Verification items for the finished model (mm, model axes). Coordinates: 2 decimals unless noted, no trailing zeros. Order: outer loops, then holes, each group sorted by start corner. A loop starts at its lowest first (then second) coordinate and runs counter-clockwise, first axis right, second up. Notation, with made-up numbers: (34.25, 63.25) - (68.25, 63.25) arc R31 ccw to (68.25, 100.25) - close; hole circle Ø3 at (71, 84). An arc over 180 degrees is marked (long way). Answer as CSV lines item,"result". Start each with the question number.
1. Material ranges on L1, parallel to Y at x = 0, z = 153.95; L2, parallel to Y at x = 10.5, z = 153.15; L3, parallel to X at y = 37, z = 152.7, recorded low to high. Write a range as [from, to].
2. Section check C-C (x = 7). Record the cut outline in (y, z), and give its area (3 significant figures).
3. Section check B-B (y = -9.5). Record the cut outline in (x, z).
4. Go/stop test with a flat-tipped pin: pin 1 (5 mm diameter, centred on x = 0, y = -41.63, fed in from -Z). Record where the tip stops, or that it passes through.
5. Section check D-D (z = 154.45). Count the separate pieces of the cut face and the enclosed holes in it, and give its area (3 significant figures).
6. Section check A-A (x = -37.5). Record the cut outline in (y, z).
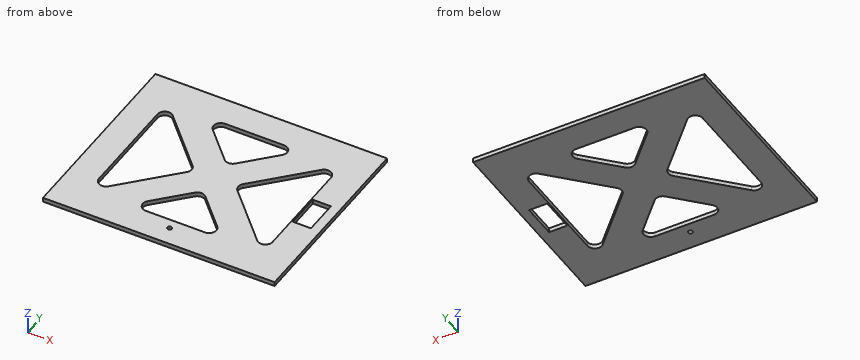
from build123d import *

# Parameters (mm, degrees)
SKETCH1_W           = 160
SKETCH1_H           = 135
BOSS_EXTRUDE1_DEPTH = 3
CUT_EXTRUDE1_DEPTH  = 20
SKETCH3_W           = 10
SKETCH3_H           = 20.2
CUT_EXTRUDE2_DEPTH  = 10
SKETCH5_W           = 10
SKETCH5_H           = 3
BOSS_EXTRUDE2_DEPTH = 30
SKETCH6_W           = 10
SKETCH6_H           = 20.15
CUT_EXTRUDE3_DEPTH  = 30
SKETCH7_W           = 10
SKETCH7_H           = 3
BOSS_EXTRUDE3_DEPTH = 30
SKETCH8_W           = 11.5
SKETCH8_H           = 21.5
CUT_EXTRUDE4_DEPTH  = 10
SKETCH9_W           = 11.5
SKETCH9_H           = 3
BOSS_EXTRUDE5_DEPTH = 30
SKETCH10_W          = 11
SKETCH10_H          = 21
CUT_EXTRUDE5_DEPTH  = 30
SKETCH11_W          = 3
SKETCH11_H          = 21
CUT_EXTRUDE6_DEPTH  = 1.5
SKETCH12_W          = 12.5
SKETCH12_H          = 3
CUT_EXTRUDE7_DEPTH  = 3


with BuildPart() as part:
    # Sketch1 → Boss-Extrude1 (new body)
    with BuildSketch(Plane.XY.offset(152)):
        with Locations((0, 12.91714511)):
            Rectangle(SKETCH1_W, SKETCH1_H)
        with BuildLine():
            Line((-60, -22.204596664), (-60, 48.038886885))
            ThreePointArc((-60, 48.038886885), (-56.872665603, 52.674954566), (-51.402750584, 51.511608676))
            Line((-51.402750584, 51.511608676), (-17.49683417, 16.389866902))
            ThreePointArc((-17.49683417, 16.389866902), (-16.094083586, 12.91714511), (-17.49683417, 9.444423319))
            Line((-17.49683417, 9.444423319), (-51.402750584, -25.677318456))
            ThreePointArc((-51.402750584, -25.677318456), (-56.872665603, -26.840664345), (-60, -22.204596664))
        make_face(mode=Mode.SUBTRACT)
        with BuildLine():
            Line((20.424315219, 60.41714511), (-20.424315219, 60.41714511))
            ThreePointArc((-20.424315219, 60.41714511), (-25.026684661, 57.371165459), (-24.021564635, 51.944423319))
            Line((-24.021564635, 51.944423319), (-3.597249416, 30.787716735))
            ThreePointArc((-3.597249416, 30.787716735), (0, 29.260438526), (3.597249416, 30.787716735))
            Line((3.597249416, 30.787716735), (24.021564635, 51.944423319))
            ThreePointArc((24.021564635, 51.944423319), (25.026684661, 57.371165459), (20.424315219, 60.41714511))
        make_face(mode=Mode.SUBTRACT)
        with BuildLine():
            Line((51.402750584, 51.511608676), (17.49683417, 16.389866902))
            ThreePointArc((17.49683417, 16.389866902), (16.094083586, 12.91714511), (17.49683417, 9.444423319))
            Line((17.49683417, 9.444423319), (51.402750584, -25.677318456))
            ThreePointArc((51.402750584, -25.677318456), (56.872665603, -26.840664345), (60, -22.204596664))
            Line((60, -22.204596664), (60, 48.038886885))
            ThreePointArc((60, 48.038886885), (56.872665603, 52.674954566), (51.402750584, 51.511608676))
        make_face(mode=Mode.SUBTRACT)
        with BuildLine():
            Line((-24.021564635, -26.110133098), (-3.597249416, -4.953426514))
            ThreePointArc((-3.597249416, -4.953426514), (0, -3.426148305), (3.597249416, -4.953426514))
            Line((3.597249416, -4.953426514), (24.021564635, -26.110133098))
            ThreePointArc((24.021564635, -26.110133098), (25.026684661, -31.536875238), (20.424315219, -34.58285489))
            Line((20.424315219, -34.58285489), (-20.424315219, -34.58285489))
            ThreePointArc((-20.424315219, -34.58285489), (-25.026684661, -31.536875238), (-24.021564635, -26.110133098))
        make_face(mode=Mode.SUBTRACT)
    extrude(amount=BOSS_EXTRUDE1_DEPTH)

    # Sketch2 → Cut-Extrude1 (cut)
    with BuildSketch(Plane.XY.offset(155)):
        with BuildLine():
            ThreePointArc((1.5, -41.631936217), (0, -40.131936217), (-1.5, -41.631936217))
            Line((-1.5, -41.631936217), (1.5, -41.631936217))
        make_face()
        with BuildLine():
            Line((1.5, -41.631936217), (-1.5, -41.631936217))
            ThreePointArc((-1.5, -41.631936217), (0, -43.131936217), (1.5, -41.631936217))
        make_face()
    extrude(amount=-CUT_EXTRUDE1_DEPTH, mode=Mode.SUBTRACT)

    # Sketch3 → Cut-Extrude2 (cut)
    with BuildSketch(Plane(origin=(80, -54.58285489, 155), x_dir=(-1, 0, 0), z_dir=(0, 0, -1))):
        with Locations((13, 65)):
            Rectangle(SKETCH3_W, SKETCH3_H)
    extrude(amount=CUT_EXTRUDE2_DEPTH, mode=Mode.SUBTRACT)

    # Sketch5 → Boss-Extrude2 (add)
    with BuildSketch(Plane(origin=(0, 0.31714511, 0), x_dir=(1, 0, 0), z_dir=(0, 1, 0))):
        with Locations((67, -153.5)):
            Rectangle(SKETCH5_W, SKETCH5_H)
    extrude(amount=BOSS_EXTRUDE2_DEPTH)

    # Sketch6 → Cut-Extrude3 (cut)
    with BuildSketch(Plane.XY.offset(155)):
        with Locations((67, 14.39214511)):
            Rectangle(SKETCH6_W, SKETCH6_H)
    extrude(amount=-CUT_EXTRUDE3_DEPTH, mode=Mode.SUBTRACT)

    # Sketch7 → Boss-Extrude3 (add)
    with BuildSketch(Plane(origin=(0, 4.31714511, 0), x_dir=(1, 0, 0), z_dir=(0, 1, 0))):
        with Locations((67, -153.5)):
            Rectangle(SKETCH7_W, SKETCH7_H)
    extrude(amount=BOSS_EXTRUDE3_DEPTH)

    # Sketch8 → Cut-Extrude4 (cut)
    with BuildSketch(Plane.XY.offset(155)):
        with Locations((73.437153805, 5.004502564)):
            Rectangle(SKETCH8_W, SKETCH8_H)
    extrude(amount=-CUT_EXTRUDE4_DEPTH, mode=Mode.SUBTRACT)

    # Sketch9 → Boss-Extrude5 (add)
    with BuildSketch(Plane(origin=(0, -5.745497436, 0), x_dir=(1, 0, 0), z_dir=(0, 1, 0))):
        with Locations((73.437153805, -153.5)):
            Rectangle(SKETCH9_W, SKETCH9_H)
    extrude(amount=BOSS_EXTRUDE5_DEPTH)

    # Sketch10 → Cut-Extrude5 (cut)
    with BuildSketch(Plane.XY.offset(155)):
        with Locations((66.5, 10.91714511)):
            Rectangle(SKETCH10_W, SKETCH10_H)
    extrude(amount=-CUT_EXTRUDE5_DEPTH, mode=Mode.SUBTRACT)

    # Sketch11 → Cut-Extrude6 (cut)
    with BuildSketch(Plane.ZY.offset(-72)):
        with Locations((153.5, 10.91714511)):
            Rectangle(SKETCH11_W, SKETCH11_H)
    extrude(amount=-CUT_EXTRUDE6_DEPTH, mode=Mode.SUBTRACT)

    # Sketch12 → Cut-Extrude7 (cut)
    with BuildSketch(Plane(origin=(0, 21.41714511, 0), x_dir=(-1, 0, 0), z_dir=(0, -1, 0))):
        with Locations((-67.25, -153.5)):
            Rectangle(SKETCH12_W, SKETCH12_H)
    extrude(amount=-CUT_EXTRUDE7_DEPTH, mode=Mode.SUBTRACT)


solid = part.part
Evaluation:
1,L1,"y = [-54.58, -43.13], [-40.13, -34.58], [-3.43, 29.26], [60.42, 80.42]"
1,L2,"y = [-54.58, -34.58], [-12.1, 37.94], [60.42, 80.42]"
1,L3,"x = [-80, -60], [-37.39, -9.59], [9.59, 37.39], [60, 80]"
2,outline,"(-54.58, 152) - (-34.58, 152) - (-34.58, 155) - (-54.58, 155) - close; (-8.48, 152) - (34.31, 152) - (34.31, 155) - (-8.48, 155) - close; (60.42, 152) - (80.42, 152) - (80.42, 155) - (60.42, 155) - close"
2,area,"248 mm²"
3,outline,"(-80, 152) - (-60, 152) - (-60, 155) - (-80, 155) - close; (-35.79, 152) - (-7.99, 152) - (-7.99, 155) - (-35.79, 155) - close; (7.99, 152) - (35.79, 152) - (35.79, 155) - (7.99, 155) - close; (60, 152) - (80, 152) - (80, 155) - (60, 155) - close"
4,pin 1,"stops at z = 152"
5,separate pieces,"1"
5,enclosed holes,"6"
5,area,"15,100 mm²"
6,outline,"(-54.58, 152) - (-11.28, 152) - (-11.28, 155) - (-54.58, 155) - close; (37.11, 152) - (80.42, 152) - (80.42, 155) - (37.11, 155) - close"
